Autodesk Inventor part; units mm, degrees
ref_plane "YZ Plane" through (0, 0, 0) normal (1, 0, 0) x (0, 1, 0)
ref_plane "XZ Plane" through (0, 0, 0) normal (0, 1, 0) x (-1, 0, 0)
ref_plane "XY Plane" through (0, 0, 0) normal (0, 0, 1) x (1, 0, 0)
sketch "Skizze1" plane through (0, 0, 0) normal (0, 0, 1) x (1, 0, 0)
  line L0 (0, 0) -> (-52.5, 0)
  arc A0 (-77.5, 25) -> (-52.5, 0) centre (-52.5, 25) ccw
  line L1 (-77.5, 25) -> (-77.5, 50)
  line L2 (-77.5, 50) -> (-72.5, 50)
  line L3 (-72.5, 50) -> (-72.5, 25)
  arc A1 (-72.5, 25) -> (-52.5, 5) centre (-52.5, 25) ccw
  line L4 (-52.5, 5) -> (0, 5)
  line L5 (0, 5) -> (0, 0)
  line L6 (-1, 5) -> (-1, 0)
  line L7 (-5, 5) -> (-5, 0)
  point P0 (-75, 50)
  dimension "d0" = 5
  dimension "d2" = 50
  dimension "d3" = 25
  dimension "d4" = 150
  dimension "d6" = 10
  dimension "d7" = 2
  dimension "d15" = 5
  dimension "d16" = 3
  dimension "d17" = 60
  dimension "d19" = 25
extrude "Extrusion1" add sketch "Skizze1" along normal blind 2
extrude "Extrusion2" add sketch "Skizze1" along normal blind 5 contours L0 L7 L4 L6
mirror "Spiegeln1" about plane through (0, 0, 0) normal (1, 0, 0) of "Extrusion1", "Extrusion2"
chamfer "Fase1" distance 3 angle 45 2 edges at (-5, 2.5, 5) (5, 2.5, 5)
properties part number "LEDholderh_3D-Druck"
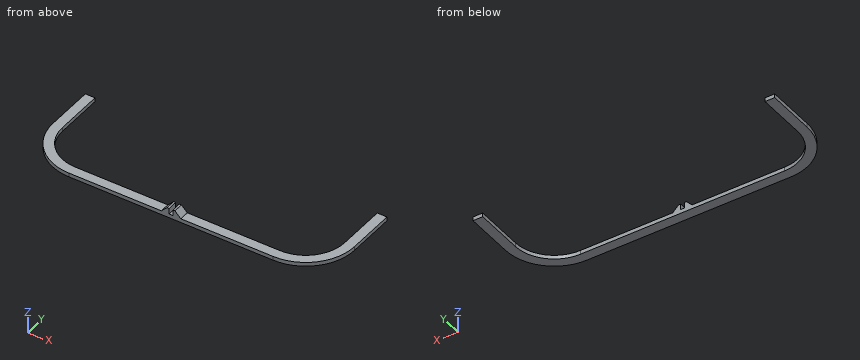
Read the model definition and answer for the solid it produces. Units are mm, in the model's axes. Round coordinates to 2 decimals unless told otherwise and drop trailing zeros. Write each loop counter-clockwise with the first axis right and the second up, starting at its lowest first coordinate (ties: lowest second). Pieces come first, ordered by that corner, then holes. Notation, with made-up numbers: (1, 17.5) -> (13, 17.5) arc R11 cw to (13, 28.5) -> close; hole circle Ø9 at (-24.75, 58.5). An arc over 180 degrees is marked (long way). Answer in a Markdown table with one row per item. Add a question column.
1) Given P1, Ø0.6, axis at x = 0, y = 3.5, coming from the +Z side; P2, Ø1.5, axis at x = -1, z = 3.5, coming from the +Y side, each flat-ended and moving along its own axis, determine where each tip first touches the part or whether it passes through.
2) Find section A-A, the plane y = 28. Determine the outline of the cut face in (x, z).
3) Find section B-B, the plane z = 3.15. Determine the outline of the cut face in (x, y), and give its area (3 significant figures).
4) Consider line 1 (X direction, y = 25.5, z = 1.85); line 2 (Z direction, x = -46.5, y = 2.5); line 3 (Y direction, x = -31.5, z = 1.9). Determine where each line is inside the solid, lowest interval first.
5) Find section C-C, the plane x = -18.5. Determine the outline of the cut face in (y, z).
Findings below:
| question | item | result |
|---|---|---|
| 1 | P1 | z = 2 |
| 1 | P2 | y = 5 |
| 2 | outline | (-77.5, 0) -> (-72.5, 0) -> (-72.5, 2) -> (-77.5, 2) -> close; (72.5, 0) -> (77.5, 0) -> (77.5, 2) -> (72.5, 2) -> close |
| 3 | outline | (-3.85, 0) -> (-1, 0) -> (-1, 5) -> (-3.85, 5) -> close; (1, 0) -> (3.85, 0) -> (3.85, 5) -> (1, 5) -> close |
| 3 | area | 28.5 mm² |
| 4 | line 1 | -77.5 to -72.5, 72.5 to 77.5 |
| 4 | line 2 | 0 to 2 |
| 4 | line 3 | 0 to 5 |
| 5 | outline | (0, 0) -> (5, 0) -> (5, 2) -> (0, 2) -> close |
